```python
from build123d import *

# Parameters (mm, degrees)
SKETCH1_W                  = 15
SKETCH1_H                  = 20
BOSS_EXTRUDE1_DEPTH        = 10
SKETCH2_W                  = 13.4
SKETCH2_H                  = 18.4
CUT_EXTRUDE1_DEPTH         = 27.925824036
CUT_EXTRUDE2_DEPTH         = 27.925824036
F_4_5_4_5_DIAMETER_HOLE1_D = 4.5
CHAMFER1_SIZE              = 2
FILLET1_R                  = 1.5
FILLET2_R                  = 3.1


with BuildPart() as part:
    # Sketch1 → Boss-Extrude1 (new body)
    with BuildSketch(Plane(origin=(10, 0, 0), x_dir=(0, 0, -1), z_dir=(1, 0, 0))):
        with Locations((7.5, 10)):
            Rectangle(SKETCH1_W, SKETCH1_H)
    extrude(amount=-BOSS_EXTRUDE1_DEPTH)

    # Sketch2 → Cut-Extrude1 (cut, through all)
    with BuildSketch(Plane.ZY):
        with Locations((-8.3, 10.8)):
            Rectangle(SKETCH2_W, SKETCH2_H)
    extrude(amount=-CUT_EXTRUDE1_DEPTH, mode=Mode.SUBTRACT)

    # Sketch3 → Cut-Extrude2 (cut, through all)
    with BuildSketch(Plane.XZ):
        with BuildLine():
            Line((7.25, -9.5), (7.25, -6.5))
            ThreePointArc((7.25, -6.5), (5, -4.25), (2.75, -6.5))
            Line((2.75, -6.5), (2.75, -9.5))
            ThreePointArc((2.75, -9.5), (5, -11.75), (7.25, -9.5))
        make_face()
    extrude(amount=-CUT_EXTRUDE2_DEPTH, mode=Mode.SUBTRACT)

    # Ø4.5 (4.5) Diameter Hole1 (through all)
    with Locations(Plane(origin=(0, 0, -1.6), x_dir=(-1, 0, 0), z_dir=(0, 0, -1))):
        with Locations((-5, 10)):
            Hole(F_4_5_4_5_DIAMETER_HOLE1_D / 2)

    # Chamfer1
    chamfer1_edges = [part.edges().sort_by_distance(p)[0] for p in [
        (0, 0.8, -15),
        (10, 20, -0.8),
        (0, 20, -0.8),
        (10, 0.8, -15),
    ]]
    chamfer(chamfer1_edges, length=CHAMFER1_SIZE)

    # Fillet1
    fillet1_edges = [part.edges().sort_by_distance(p)[0] for p in [
        (5, 1.6, -1.6),
    ]]
    fillet(fillet1_edges, radius=FILLET1_R)

    # Fillet2
    fillet2_edges = [part.edges().sort_by_distance(p)[0] for p in [
        (5, 0, 0),
    ]]
    fillet(fillet2_edges, radius=FILLET2_R)


solid = part.part
```
Could you check a few things on this model? Use its own coordinates, in mm. A direction names the side the tool comes from. Coordinates: 2 decimals unless noted, no trailing zeros. Write each loop counter-clockwise with the first axis right and the second up, starting at its lowest first coordinate (ties: lowest second). Pieces come first, ordered by that corner, then holes. Notation, with made-up numbers: M 39.25,-18.75 L 95.25,-18.75 A29 ccw 95.25,11.25 Z; hole C -17,66.25 d7. An arc over 180 degrees is marked long. Answer as CSV lines item,"result". Start each with the question number.
1) For faces 1 (the flat face through (2.75, 1, -8)), 2 (the flat face through (1, 1, -14)), which set-ups out of +Z, -Z, +X, -X, +Y, -Y let a thin tool reach every point of the face, with its end or its side?
2) We'd pull the mould along X, two halves only. Please class faces 3 (the cylindrical face through (5.05, 0.79, -4.25)), 4 (the flat face through (5, 13, -1.6)), 5 (the flat face through (9, 19, -1)): +X half, -X half, draft (parallel to the pull), parting line (faces both ways), or undercut.
3) Please list where these lines run through material, in increasing order: line 1 (Y direction, x = 8.5, z = -7.5); line 2 (Z direction, x = 2, y = 17); line 3 (Y direction, x = 5, z = -1). Write a range as from..to.
4) I want a section at A-A, the plane x = 5. Please give me the cut outline in (y, z).
5) I want a section at D-D, the plane x = 2.5. Please give me the cut outline in (y, z), and give its area (3 significant figures).
6) I want a section at C-C, the plane y = 10. Please give me the cut outline in (x, z), and give its area (3 significant figures).
7) I want a section at B-B, the plane z = -5. Please give me the cut outline in (x, y).
8) For P1, Ø5, axis at x = 3.5, z = -10.5, coming from the +Y side; P2, Ø3, axis at x = 6, y = 15, coming from the -Z side, each with a flat end and sliding along its axis, tell me the tip position at first contact or that it passes through.
Data:
1,face 1,"+Y, -Y"
1,face 2,"-Z, -X, +Y, -Y"
2,face 3,"undercut"
2,face 4,"draft"
2,face 5,"+X half"
3,line 1,"y = 0..1.6"
3,line 2,"z = -1.6..0"
3,line 3,"y = 0.82..7.75, 12.25..20"
4,outline,"M 0,-15 L 1.6,-15 L 1.6,-11.75 L 0,-11.75 Z; M 0,-4.25 L 1.6,-4.25 L 1.6,-3.1 A1.5 cw 3.1,-1.6 L 7.75,-1.6 L 7.75,0 L 3.1,0 A3.1 ccw 0,-3.1 Z; M 12.25,-1.6 L 20,-1.6 L 20,0 L 12.25,0 Z"
5,outline,"M 0,-15 L 1.6,-15 L 1.6,-3.1 A1.5 cw 3.1,-1.6 L 20,-1.6 L 20,0 L 3.1,0 A3.1 ccw 0,-3.1 Z"
5,area,"51.9 mm^2"
6,outline,"M 0,-1.6 L 2.75,-1.6 L 2.75,0 L 0,0 Z; M 7.25,-1.6 L 10,-1.6 L 10,0 L 7.25,0 Z"
6,area,"8.80 mm^2"
7,outline,"M 0,0 L 3.32,0 L 3.32,1.6 L 0,1.6 Z; M 6.68,0 L 10,0 L 10,1.6 L 6.68,1.6 Z"
8,P1,"stops at y = 1.6"
8,P2,"stops at z = -1.6"
